Input: dimensioned drawing with shaded views. Units: mm. Origin: part minimum x, y, z. Round coordinates to 2 decimals unless told otherwise and drop trailing zeros. Order: outer loops, then holes, each group sorted by start corner. A loop starts at its lowest first (then second) coordinate and runs counter-clockwise, first axis right, second up. Notation, with made-up numbers: (62, 10.25) - (71, 10.25) arc R18 ccw to (71, 36.25) - close; hole circle Ø9 at (4, -24). An arc over 180 degrees is marked (long way). One line per item, written item: value. Start each with the question number.
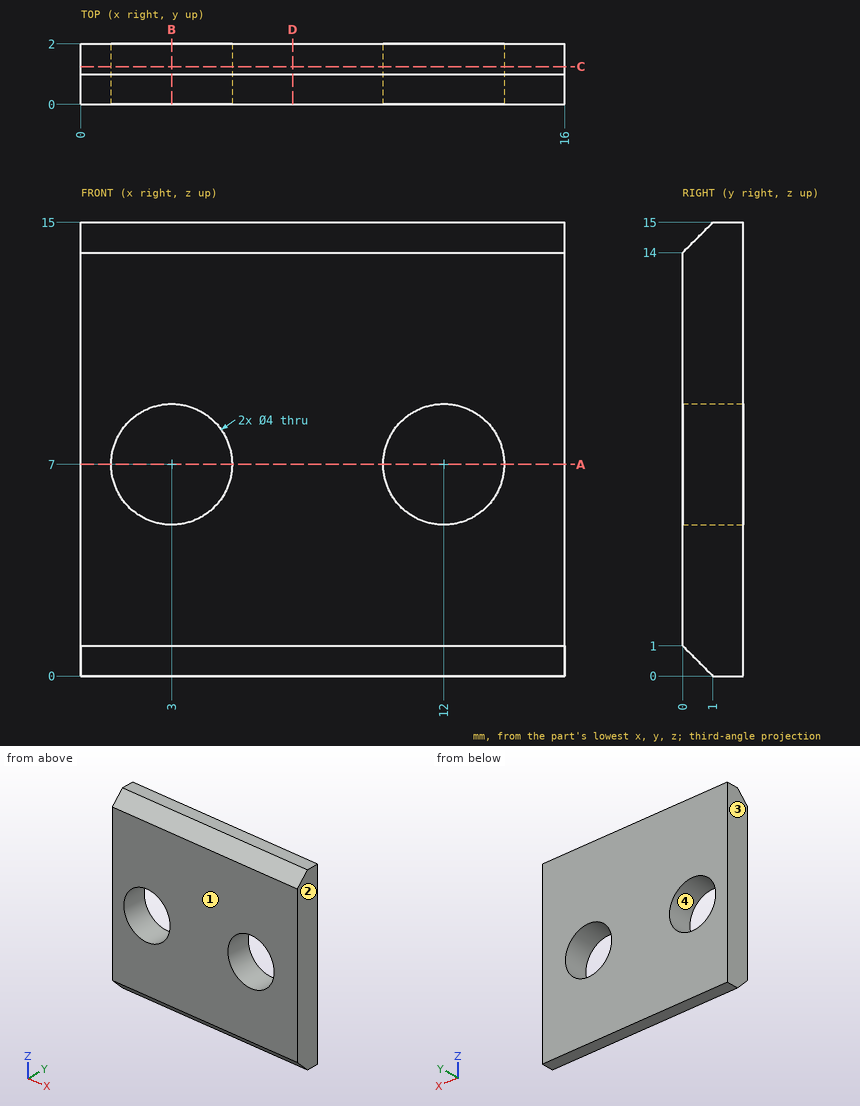
1. Section A-A (z = 7). Return the cut outline in (x, y).
2. Line query: line 1 (X direction, y = 0.95, z = 6); line 2 (Z direction, x = 12, y = 1.2); line 3 (Z direction, x = 12, y = 0.8). Output: solid intervals per line, ascending. Write a range as from..to.
3. Section C-C (y = 1.25). Return the cut outline in (x, z).
4. Pin query (flat end, axial travel): pin 1 (2.5 mm diameter, centred on x = 3, z = 7, fed in from +Y). Return the tip coordinate at first contact, or that it passes through.
5. Pull-direction query (X, two-part tool) for the marked faces 1, 2, 3 and 4; classes: released by +X, released by -X, zero draft, split by the parting line, or undercut.
6. Section B-B (x = 3). Return the cut outline in (y, z), then the cut area to 3 significant figures.
7. Section D-D (x = 7). Return the cut outline in (y, z), then the cut area to 3 significant figures.
Solved:
1. outline: (0, 0) - (1, 0) - (1, 2) - (0, 2) - close; (5, 0) - (10, 0) - (10, 2) - (5, 2) - close; (14, 0) - (16, 0) - (16, 2) - (14, 2) - close
2. line 1: x = 0..1.27, 4.73..10.27, 13.73..16
2. line 2: z = 0..5, 9..15
2. line 3: z = 0.2..5, 9..14.8
3. outline: (0, 0) - (16, 0) - (16, 15) - (0, 15) - close; hole circle Ø4 at (3, 7); hole circle Ø4 at (12, 7)
4. pin 1: passes through
5. face 1: zero draft
5. face 2: released by +X
5. face 3: released by -X
5. face 4: undercut
6. outline: (0, 1) - (1, 0) - (2, 0) - (2, 5) - (0, 5) - close; (0, 9) - (2, 9) - (2, 15) - (1, 15) - (0, 14) - close
6. area: 21.0 mm²
7. outline: (0, 1) - (1, 0) - (2, 0) - (2, 15) - (1, 15) - (0, 14) - close
7. area: 29.0 mm²
